Verification items for the finished model (mm, model axes). A direction names the side the tool comes from. Round coordinates to 2 decimals unless told otherwise and drop trailing zeros. Write each loop counter-clockwise with the first axis right and the second up, starting at its lowest first coordinate (ties: lowest second). Pieces come first, ordered by that corner, then holes. Notation, with made-up numbers: M 80.25,38.25 L 108.25,38.25 A18 cw 108.25,69.25 Z; hole C 4.25,88.5 d8. An arc over 180 degrees is marked long. Write each question's results on one line, items separated by ' | '.
from build123d import *

# Parameters (mm, degrees)
F2_R            = 2.25
F3_DEPTH        = 28
F3_COPIES_COUNT = 4


# Not quite as in the source:
# - a pattern or mirror of a feature is missing from the dataset's text; its kind, count and spacing are read off the source's solid


with BuildPart() as f1:
    # F0 (on Front) → F1 (revolve)
    with BuildSketch(Plane.XZ):
        Polygon((26.1, 27.5), (17.25, 27.5), (17.25, 2.5), (17.25, -2.5), (21.1, -2.5), (21.1, -37.5), (26.1, -37.5), align=None)
    revolve(axis=Axis((0, 0, 0), (0, 0, -1)))

    # F2 (on Front) → F3 (cut)
    with BuildSketch(Plane.XZ):
        with Locations((0, 14.8)):
            Circle(F2_R)
        with Locations((0, -22.5)):
            Circle(F2_R)
    f3 = extrude(amount=-F3_DEPTH, mode=Mode.SUBTRACT)

    # F3_copies: F3 ×4 about axis
    f3_copies_axis = Axis((0, 0, 0), (0, 0, 1))
    for i in range(1, F3_COPIES_COUNT):
        add(f3.rotate(f3_copies_axis, i * 360 / F3_COPIES_COUNT), mode=Mode.SUBTRACT)


solid = f1.part
1) Sectioned sample at A-A, the plane x = 0. Record the cut outline in (y, z), and give its area (3 significant figures).
Calculated:
outline: M -26.1,-37.5 L -21.1,-37.5 L -21.1,-24.75 L -26.1,-24.75 Z; M -26.1,-20.25 L -21.1,-20.25 L -21.1,-2.5 L -17.25,-2.5 L -17.25,12.55 L -26.1,12.55 Z; M -26.1,17.05 L -17.25,17.05 L -17.25,27.5 L -26.1,27.5 Z; M 17.25,-2.5 L 21.1,-2.5 L 21.1,-20.25 L 26.1,-20.25 L 26.1,12.55 L 17.25,12.55 Z; M 17.25,17.05 L 26.1,17.05 L 26.1,27.5 L 17.25,27.5 Z; M 21.1,-37.5 L 26.1,-37.5 L 26.1,-24.75 L 21.1,-24.75 Z | area: 756 mm²
2) Depth check by flat-ended pin: P1, Ø3.5, axis at x = 0, z = 14.8, coming from the -Y side; P2, Ø5, axis at x = 12.5, z = -30.5, coming from the +Y side; P3, Ø6, axis at y = 9, z = -20, coming from the -X side; P4, Ø6, axis at y = 14.5, z = 9, coming from the -X side. Enter the tip coordinate at first touch or a pass-through.
Calculated:
P1: passes through | P2: stops at y = 24.11 | P3: stops at x = -25.4 | P4: stops at x = -23.43
3) Draft check along Z on faces 3 (the flat face through (17, 5, 27.5)), 4 (the cylindrical face through (0.488, -23.504, -24.696)), 5 (the flat face through (-10, 19, -37.5)). Enter one of: pulls with the +Z half, pulls with the -Z half, needs draft (parallel to the pull), parting line crosses it, or undercut.
Calculated:
face 3: pulls with the +Z half | face 4: undercut | face 5: pulls with the -Z half
4) Sectioned sample at D-D, the plane z = -22.5. Record the cut outline in (x, y).
Calculated:
outline: M -26,-2.25 A26.1 ccw -2.25,-26 L -2.25,-20.98 A21.1 cw -20.98,-2.25 Z; M -26,2.25 L -20.98,2.25 A21.1 cw -2.25,20.98 L -2.25,26 A26.1 ccw Z; M 2.25,-26 A26.1 ccw 26,-2.25 L 20.98,-2.25 A21.1 cw 2.25,-20.98 Z; M 2.25,20.98 A21.1 cw 20.98,2.25 L 26,2.25 A26.1 ccw 2.25,26 Z
5) Access from +Z, -Z, +X, -X, +Y, -Y to the whole of each face (thin tool, end or side, straight path). Record for faces 1 (the cylindrical face through (-21.538, -0.488, 12.604)), 2 (the flat face through (8, 16, -2.5)).
Calculated:
face 1: +X, -X | face 2: -Z
6) Sectioned sample at C-C, the plane x = -10. Record the cut outline in (y, z), and give its area (3 significant figures).
Calculated:
outline: M -24.11,-37.5 L -18.58,-37.5 L -18.58,-2.5 L -14.06,-2.5 L -14.06,27.5 L -24.11,27.5 Z; M 14.06,-2.5 L 18.58,-2.5 L 18.58,-37.5 L 24.11,-37.5 L 24.11,27.5 L 14.06,27.5 Z | area: 990 mm²
7) Sectioned sample at B-B, the plane y = 15. Record the cut outline in (x, z).
Calculated:
outline: M -21.36,-37.5 L -14.84,-37.5 L -14.84,-2.5 L -8.52,-2.5 L -8.52,27.5 L -21.36,27.5 Z; M 8.52,-2.5 L 14.84,-2.5 L 14.84,-37.5 L 21.36,-37.5 L 21.36,27.5 L 8.52,27.5 Z
8) Material ranges on line 1 (Z direction, x = 22, y = 0); line 2 (Z direction, x = 1, y = -22); line 3 (Z direction, x = 0, y = -21), recorded low to high. Write a range as [from, to].
Calculated:
line 1: z = [-37.5, -24.75], [-20.25, 12.55], [17.05, 27.5] | line 2: z = [-37.5, -24.52], [-20.48, 12.78], [16.82, 27.5] | line 3: z = [-2.5, 12.55], [17.05, 27.5]
